Input: part model. Units: mm. Frame: model coordinates. Face numbers are marked on the shaded views. A direction names the side the tool comes from. Give positions to 0.01 mm unless a question says otherwise; leave off trailing zeros. Loops run counter-clockwise (first coordinate to the right, second up) from the corner with the lowest first, then second, coordinate; pieces in that order, holes last. Notation, with made-up numbers: M -1,-33.5 L 4,-33.5 A29 cw 4,-11.5 Z; hole C 54,46.25 d5. An arc over 180 degrees is marked long. Use CSV: the item, a comma, the result in double quotes. Start each with the question number.
Q1. Pin query (flat end, axial travel): pin 1 (1 mm diameter, centred on x = 0, z = -55.5, fed in from +Y); pin 2 (8 mm diameter, centred on y = -4.5, z = -29.5, fed in from -X); pin 3 (4 mm diameter, centred on x = -3, z = -24, fed in from +Y); pin 4 (6 mm diameter, centred on x = -1, z = -17.5, fed in from +Y). Return the tip coordinate at first contact, or that it passes through.
Q2. Section D-D, the plane y = -21. Output: boundary loops of the cut face in (x, z).
Q3. Pull-direction query (Y, two-part tool) for the marked faces 1, 2 and 3; classes: released by +Y, released by -Y, zero draft, split by the parting line, or undercut.
Q4. Material intervals for line 1 along Z through (x, y) = (-7.75, -19.5); line 2 along Y through (x, z) = (2.25, -68.5); line 3 along Y through (x, z) = (4.25, -61.5), sorted ascending.
Q5. Section C-C, the plane x = 4.5. Output: boundary loops of the cut face in (y, z), plus the area to 3 significant figures.
Q6. Section B-B, the plane y = -10. Output: boundary loops of the cut face in (x, z).
Q7. Section A-A, the plane z = 0. Output: boundary loops of the cut face in (x, y).
Q8. Reachability of the marked faces 4, 5 and 6 from +Z, -Z, +X, -X, +Y, -Y: full face, straight path, thin tool, end or side. Return the list, or none.
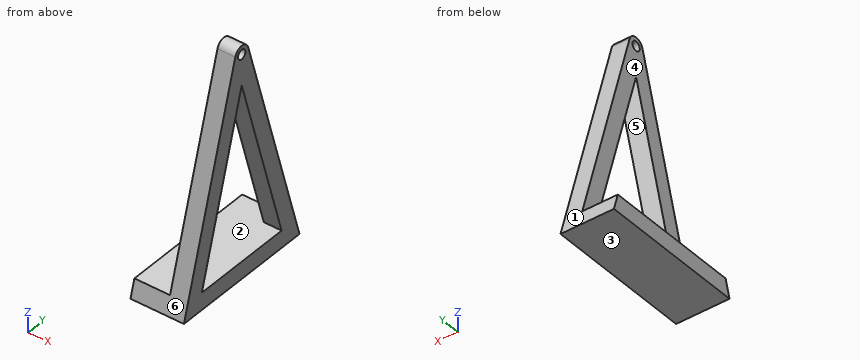
Autodesk Inventor part; units mm, degrees
ref_plane "YZ Plane" through (0, 0, 0) normal (1, 0, 0) x (0, 1, 0)
ref_plane "XZ Plane" through (0, 0, 0) normal (0, 1, 0) x (-1, 0, 0)
ref_plane "XY Plane" through (0, 0, 0) normal (0, 0, 1) x (1, 0, 0)
sketch "Sketch1" plane through (0, 0, 0) normal (1, 0, 0) x (0, 1, 0)
  circle A0 centre (0, 0) radius 2.9
  line L0 (-2.783, 0.8155) -> (-25, -75)
  line L1 (25, -75) -> (2.783, 0.8155)
  line L2 (52.7128, 0) -> (52.7128, -59)
  line L3 (52.7128, -59) -> (25, -75)
  line L4 (-40.5426, 0) -> (68.2554, 0)
  line L5 (17.2565, -69.2) -> (0, -10.3124)
  line L6 (0, -10.3124) -> (-17.2565, -69.2)
  line L7 (-17.2565, -69.2) -> (17.2565, -69.2)
  line L8 (0, -90.58) -> (0, 18.48)
  line L9 (25, -75) -> (-25, -75)
  dimension "d0" = 5.8
  dimension "d1" = 32
  dimension "d4" = 30
  dimension "d19" = 5.8
  dimension "d20" = 50
  dimension "d21" = 75
extrude "Extrusion1" add sketch "Sketch1" along normal blind 6 contours L4 L8 A0 | L4 L1 L9 L8 L7 L5 A0 | A0 L8 L4 | A0 L1 L4 | L8 L6 L7 L9 L0 L4 A0 | A0 L4 L8 | L4 A0 L8 | L4 L0 A0
hole "Hole1" at (0, 0, 0) direction (1, 0, 0) diameter 3.2 end through all
sketch "Sketch3" plane through (0, 0, 0) normal (-1, 0, 0) x (0, 0, 1)
  line L0 (-75, 25) -> (0.8155, 2.783)
  line L1 (-75, -25) -> (-75, 25)
  line L2 (0.8155, -2.783) -> (-75, -25)
  line L3 (-10.3124, 0) -> (-69.2, 17.2565)
  line L4 (-69.2, -17.2565) -> (-10.3124, 0)
  line L5 (-69.2, 17.2565) -> (-69.2, -17.2565)
  line L6 (-10.3124, 0) -> (-69.2, 17.2565)
  line L7 (-69.2, 17.2565) -> (-69.2, 23.3004)
  line L8 (-75, 25) -> (0.8155, 2.783)
  line L9 (-69.2, 17.2565) -> (-69.2, -17.2565)
  line L10 (-69.2, -17.2565) -> (-69.2, -23.3004)
  line L11 (0.8155, -2.783) -> (-75, -25)
  arc A0 (0.8155, -2.783) -> (0.8155, 2.783) centre (0, 0) ccw
  point P0 (0.1794, -3.245)
  point P1 (0.1794, 3.245)
  point P2 (-69.2, -23.3004)
  point P3 (-69.2, 23.3004)
extrude "Extrusion2" add sketch "Sketch3" along normal blind 12 contours L0 L7 L5 L10 L2 L1
properties part number "ArrayBracketSupport"
A:
1,pin 1,"y = 19.43"
1,pin 2,"x = 0"
1,pin 3,"through"
1,pin 4,"y = 8.98"
2,outline,"M -12,-75 L 6,-75 L 6,-61.35 L 0,-61.35 L 0,-69.2 L -12,-69.2 Z"
3,face 1,"released by +Y"
3,face 2,"undercut"
3,face 3,"zero draft"
4,line 1,"-75 to -69.2"
4,line 2,"-23.1 to -17.05, 17.05 to 23.1"
4,line 3,"-21.04 to -15, 15 to 21.04"
5,outline,"M -25,-75 L 25,-75 L 2.78,0.82 A2.9 ccw -2.78,0.82 Z; hole M -17.26,-69.2 L 17.26,-69.2 L 0,-10.31 Z; hole C 0,0 d3.2"
5,area,"1,090 mm^2"
6,outline,"M -12,-75 L 6,-75 L 6,-69.2 L -12,-69.2 Z; M 0,-44.44 L 6,-44.44 L 6,-23.81 L 0,-23.81 Z"
7,outline,"M 0,-3.02 L 6,-3.02 L 6,-1.6 L 0,-1.6 Z; M 0,1.6 L 6,1.6 L 6,3.02 L 0,3.02 Z"
8,face 4,"+Z, -X, +Y, -Y"
8,face 5,"+X, -X"
8,face 6,"+Z, +X, -X, -Y"
